Geometry: final body of the model. Coordinates: model frame, mm. Face numbers are marked on the shaded views. A direction names the side the tool comes from. Round coordinates to 2 decimals unless told otherwise and drop trailing zeros. Write each loop counter-clockwise with the first axis right and the second up, starting at its lowest first coordinate (ties: lowest second). Pieces come first, ordered by that corner, then holes.
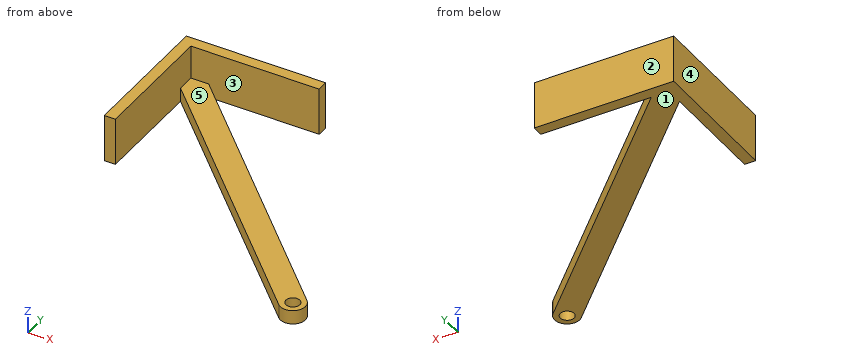
from build123d import *

# Parameters (mm, degrees)
F1_DEPTH = 5
F3_DEPTH = 12
F4_R     = 2.5
F5_DEPTH = 25


with BuildPart() as f1:
    # F0 (on Top) → F1 (new body)
    with BuildSketch(Plane.XY):
        with BuildLine():
            Line((-92.9, 92.9), (-92.9, 42.9))
            Line((-92.9, 42.9), (-88.9, 42.9))
            Line((-88.9, 42.9), (-88.9, 82.536039))
            Line((-88.9, 82.536039), (-3.181981, -3.181981))
            ThreePointArc((-3.181981, -3.181981), (3.181981, -3.181981), (3.181981, 3.181981))
            Line((3.181981, 3.181981), (-82.536039, 88.9))
            Line((-82.536039, 88.9), (-42.9, 88.9))
            Line((-42.9, 88.9), (-42.9, 92.9))
            Line((-42.9, 92.9), (-92.9, 92.9))
        make_face()
    extrude(amount=F1_DEPTH)

    # F2 (on face) → F3 (join)
    with BuildSketch(Plane.XY.offset(5)):
        Polygon((-42.9, 92.9), (-92.9, 92.9), (-92.9, 42.9), (-88.9, 42.9), (-88.9, 88.9), (-42.9, 88.9), align=None)
    extrude(amount=F3_DEPTH)

    # F4 (on face) → F5 (cut)
    with BuildSketch(Plane.XY.offset(5)):
        Circle(F4_R)
    extrude(amount=-F5_DEPTH, mode=Mode.SUBTRACT)


solid = f1.part
1) First-contact query: P1, Ø4.5, axis at y = 91.5, z = 5, coming from the +X side; P2, Ø2, axis at x = -90.5, z = 8, coming from the -Y side; P3, Ø10, axis at y = 22.5, z = 6, coming from the +X side; P4, Ø8, axis at y = 7, z = 12, coming from the +X side. Flat tips, straight axial feed; report the tip coordinate or a pass-through.
2) Line query: probe 1 along X at (y, z) = (75.5, 12); probe 2 along Y at (x, z) = (-66.5, 9.75); probe 3 along Z at (x, y) = (-80, 81). Output: solid intervals per line, ascending.
3) Section A-A on z = 1.5. Output: boundary loops of the cut face in (x, y).
4) Section D-D on z = 10.25. Output: boundary loops of the cut face in (x, y).
5) Draft query along Y for the marked faces 1, 2 and 3. Return one class per face: pulls with the +Y half, pulls with the -Y half, needs draft (parallel to the pull), parting line crosses it, or undercut.
6) Section C-C on y = 0. Output: boundary loops of the cut face in (x, z).
7) Section B-B on x = -61.5. Output: boundary loops of the cut face in (y, z).
8) Reachability of the marked faces 4 and 5 from +Z, -Z, +X, -X, +Y, -Y: full face, straight path, thin tool, end or side. Return the list, or none.
Filled in:
1. P1: stops at x = -42.9
1. P2: stops at y = 42.9
1. P3: stops at x = -11.24
1. P4: passes through
2. probe 1: x = -92.9 to -88.9
2. probe 2: y = 88.9 to 92.9
2. probe 3: z = 0 to 5
3. outline: (-92.9, 42.9) - (-88.9, 42.9) - (-88.9, 82.54) - (-3.18, -3.18) arc R4.5 ccw to (3.18, 3.18) - (-82.54, 88.9) - (-42.9, 88.9) - (-42.9, 92.9) - (-92.9, 92.9) - close; hole circle Ø5 at (0, 0)
4. outline: (-92.9, 42.9) - (-88.9, 42.9) - (-88.9, 88.9) - (-42.9, 88.9) - (-42.9, 92.9) - (-92.9, 92.9) - close
5. face 1: needs draft
5. face 2: pulls with the +Y half
5. face 3: undercut
6. outline: (-6.36, 0) - (-2.5, 0) - (-2.5, 5) - (-6.36, 5) - close; (2.5, 0) - (4.5, 0) - (4.5, 5) - (2.5, 5) - close
7. outline: (55.14, 0) - (67.86, 0) - (67.86, 5) - (55.14, 5) - close; (88.9, 0) - (92.9, 0) - (92.9, 17) - (88.9, 17) - close
8. face 4: +Z, -Z, -X, +Y, -Y
8. face 5: +Z, +X, -Y
